Verification items for the finished model (mm, model axes). A direction names the side the tool comes from. Round coordinates to 2 decimals unless told otherwise and drop trailing zeros. Loops run counter-clockwise (first coordinate to the right, second up) from the corner with the lowest first, then second, coordinate; pieces in that order, holes last. Notation, with made-up numbers: (24, -16) -> (58, -16) arc R23 cw to (58, 5) -> close; hole circle Ø10 at (22, 46). An arc over 180 degrees is marked (long way). Use a Markdown table: item, result. Add a question column.
```python
from build123d import *

# Parameters (mm, degrees)
SKETCH1_R           = 4
BOSS_EXTRUDE1_DEPTH = 5
SKETCH2_R           = 2.5
CUT_EXTRUDE1_DEPTH  = 6
SKETCH3_R           = 2.5
BOSS_EXTRUDE2_DEPTH = 3.6
SKETCH4_R           = 2.5
BOSS_EXTRUDE3_DEPTH = 25


with BuildPart() as part:
    # Sketch1 → Boss-Extrude1 (new body)
    with BuildSketch(Plane.XY):
        with BuildLine():
            Line((0, 0), (0, 68.543560763))
            Line((0, 68.543560763), (10, 68.543560763))
            Line((10, 68.543560763), (10, 0))
            ThreePointArc((10, 0), (5, -23.956439237), (0, 0))
        make_face()
        with Locations((5, -11.456439237)):
            Circle(SKETCH1_R, mode=Mode.SUBTRACT)
    extrude(amount=BOSS_EXTRUDE1_DEPTH)

    # Sketch2 → Cut-Extrude1 (cut, through all)
    with BuildSketch(Plane.XY.offset(5)):
        with Locations((5, 63.543560763)):
            Circle(SKETCH2_R)
    extrude(amount=-CUT_EXTRUDE1_DEPTH, mode=Mode.SUBTRACT)

    # Sketch3 → Boss-Extrude2 (add)
    with BuildSketch(Plane.XY.offset(5)):
        with Locations((5, 36.043560763)):
            Circle(SKETCH3_R)
    extrude(amount=BOSS_EXTRUDE2_DEPTH)

    # Sketch4 → Boss-Extrude3 (add)
    with BuildSketch(Plane(origin=(0, 0, 0), x_dir=(-1, 0, 0), z_dir=(0, 0, -1))):
        with Locations((-5, 36.043560763)):
            Circle(SKETCH4_R)
    extrude(amount=BOSS_EXTRUDE3_DEPTH)


solid = part.part
```
1) Sectioned sample at D-D on x = 14.5. Enter the section's corners in (y, z).
2) Sectioned sample at B-B on y = 49. Enter the section's corners in (x, z), then the cut area to 3 significant figures.
3) Sectioned sample at A-A on x = 5. Enter the section's corners in (y, z).
4) Access from +Z, -Z, +X, -X, +Y, -Y to the whole of each face (thin tool, end or side, straight path). Record for faces 1 (the face through (4.48, -7.49, 2.46)), 2 (the face through (5.542, 33.603, -12.325)), 3 (the face through (0, 34, 2)), 4 (the face through (10, 35, 2)).
5) Release check for a two-part mould opening along X. For faces 5 (the face through (4.458, 33.603, 6.775)), 6 (the face through (4.458, 61.103, 2.535)), 7 (the face through (5, 36, 8.6)) record: released by +X, released by -X, zero draft, split by the parting line, or undercut.
6) Sectioned sample at C-C on z = -4. Enter the section's corners in (x, y).
7) Thickness scan on line 1 (Y direction, x = 5, z = 1.6); line 2 (Y direction, x = 7.25, z = 4.5); line 3 (Z direction, x = 8.5, y = 50.5). Record the ranges inside material, lowest first.
8) Go/stop test with flat-tipped pins: pin 1 (2.5 mm diameter, centred on y = 32, z = 1.5, fed in from -X); pin 2 (12.5 mm diameter, centred on x = 5, y = 23, fed in from -Z); pin 3 (8 mm diameter, centred on x = 10.5, z = -18, fed in from -Y). Record where each tip stops, or that it passes through.
Geometry results:
| question | item | result |
|---|---|---|
| 1 | outline | (-19.58, 0) -> (-3.33, 0) -> (-3.33, 5) -> (-19.58, 5) -> close |
| 2 | outline | (0, 0) -> (10, 0) -> (10, 5) -> (0, 5) -> close |
| 2 | area | 50.0 mm^2 |
| 3 | outline | (-23.96, 0) -> (-15.46, 0) -> (-15.46, 5) -> (-23.96, 5) -> close; (-7.46, 0) -> (33.54, 0) -> (33.54, -25) -> (38.54, -25) -> (38.54, 0) -> (61.04, 0) -> (61.04, 5) -> (38.54, 5) -> (38.54, 8.6) -> (33.54, 8.6) -> (33.54, 5) -> (-7.46, 5) -> close; (66.04, 0) -> (68.54, 0) -> (68.54, 5) -> (66.04, 5) -> close |
| 4 | face 1 | +Z, -Z |
| 4 | face 2 | -Z |
| 4 | face 3 | +Z, -Z, -X, +Y |
| 4 | face 4 | +Z, -Z, +X, +Y |
| 5 | face 5 | split by the parting line |
| 5 | face 6 | undercut |
| 5 | face 7 | zero draft |
| 6 | outline | circle Ø5 at (5, 36.04) |
| 7 | line 1 | -23.96 to -15.46, -7.46 to 61.04, 66.04 to 68.54 |
| 7 | line 2 | -23.75 to -14.76, -8.15 to 62.45, 64.63 to 68.54 |
| 7 | line 3 | 0 to 5 |
| 8 | pin 1 | x = 0 |
| 8 | pin 2 | z = 0 |
| 8 | pin 3 | y = 34.04 |
